Source: three-view drawing plus pictorial views. Frame: mm from the lowest corner of the part. Round coordinates to 2 decimals unless told otherwise and drop trailing zeros. Loops run counter-clockwise (first coordinate to the right, second up) from the corner with the lowest first, then second, coordinate; pieces in that order, holes last. Notation, with made-up numbers: M 57.5,63.5 L 95.5,63.5 A32 ccw 95.5,90.5 Z; hole C 20,5.25 d4. An arc over 180 degrees is marked long. Write each question's results on one line, items separated by ' | '.
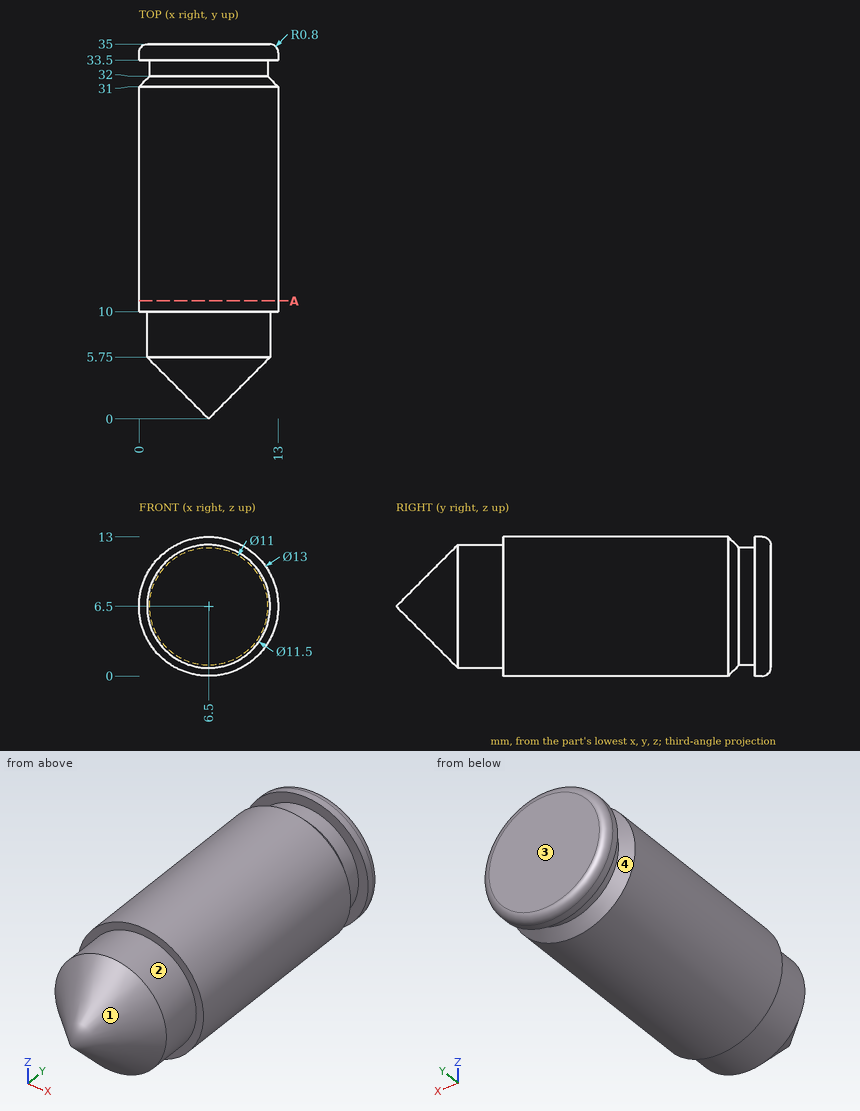
1. Pin query (flat end, axial travel): P1, Ø4, axis at x = 9.5, y = 21.5, coming from the -Z side; P2, Ø3, axis at x = 7.5, z = 2, coming from the -Y side; P3, Ø1, axis at y = 17.5, z = 11.5, coming from the -X side. Return the tip coordinate at first contact, or that it passes through.
Answer key:
P1: stops at z = 0.08 | P2: stops at y = 3.11 | P3: stops at x = 1.81
2. Ray query, probe 1 along Y at (x, z) = (10.5, 2.25); probe 2 along Z at (x, y) = (6.25, 32.5); probe 3 along X at (y, z) = (13.5, 2). Return the intervals inside material, ascending.
Answer key:
probe 1: y = 10 to 31.66, 33.5 to 34.99 | probe 2: z = 1.01 to 11.99 | probe 3: x = 1.81 to 11.19
3. Section A-A (y = 11). Output: boundary loops of the cut face in (x, z).
Answer key:
outline: C 6.5,6.5 d13
4. Draft query along Y for the marked faces 1, 2, 3 and 4. Return one class per face: pulls with the +Y half, pulls with the -Y half, needs draft (parallel to the pull), parting line crosses it, or undercut.
Answer key:
face 1: pulls with the -Y half | face 2: needs draft | face 3: pulls with the +Y half | face 4: undercut
